Part model, mm, in its own coordinate system. Face numbers are marked on the shaded views. A direction names the side the tool comes from. Give positions to 0.01 mm unless a question says otherwise; leave off trailing zeros. Order: outer loops, then holes, each group sorted by start corner. A loop starts at its lowest first (then second) coordinate and runs counter-clockwise, first axis right, second up.
1. Mould opens along X. For the marked faces 1, 2 and 3 say: +X half, -X half, draft (parallel to the pull), parting line (faces both ways), or undercut.
2. Probe line 1 (Z direction, x = 16.5, y = 2); line 2 (X direction, y = 6, z = 0.2); line 3 (Y direction, x = 28, z = 0.1). List the from-to ranges inside material, lowest first.
3. Slice it at D-D on x = 27. List the corners of the cut face in (y, z), and give its area (3 significant figures).
4. Slice it at C-C on x = 4.5. List the corners of the cut face in (y, z).
5. Slice it at B-B on z = 0.1. List the corners of the cut face in (x, y), and give its area (3 significant figures).
6. Slice it at A-A on x = -10. List the corners of the cut face in (y, z).
7. Which spindle directions (+Z, -Z, +X, -X, +Y, -Y) get a long thin tool onto all of the face, cutting with end or side? Do the marked faces 4 and 5. Say none if no direction does.
Autodesk Inventor part; units mm, degrees
ref_plane "aluschild_XY" through (0, 0, 0) normal (0, 0, 1) x (1, 0, 0)
ref_plane "aluschild_YZ" through (0, 0, 0) normal (1, 0, 0) x (0, 1, 0)
ref_plane "aluschild_ZX" through (0, 0, 0) normal (0, 1, 0) x (0, 0, 1)
sketch "Sketch_1" plane through (0, 0, 0) normal (0, 0, 1) x (1, 0, 0)
  arc A0 (-32, 0) -> (-24, -8) centre (-24, 0) ccw
  line L0 (-24, -8) -> (24, -8)
  arc A1 (24, -8) -> (32, 0) centre (24, 0) ccw
  arc A2 (32, 0) -> (24, 8) centre (24, 0) ccw
  line L1 (24, 8) -> (-24, 8)
  arc A3 (-24, 8) -> (-32, 0) centre (-24, 0) ccw
extrude "Extrusion1" add sketch "Sketch_1" along normal blind 0.3
sketch "Sketch_13" plane through (0, 0, 0.3) normal (0, 0, 1) x (1, 0, 0)
  line L0 (-12.9184, 3.0554) -> (-12.9184, -3.0496)
  line L1 (-12.9184, -3.0496) -> (-10.8856, -3.0496)
  line L2 (-10.8856, -3.0496) -> (-10.8856, -0.7401)
  line L3 (-10.8856, -0.7401) -> (-8.6487, -0.7401)
  line L4 (-8.6487, -0.7401) -> (-8.6487, -3.0496)
  line L5 (-8.6487, -3.0496) -> (-6.6154, -3.0496)
  line L6 (-6.6154, -3.0496) -> (-6.6154, 3.0554)
  line L7 (-6.6154, 3.0554) -> (-8.6487, 3.0554)
  line L8 (-8.6487, 3.0554) -> (-8.6487, 0.8356)
  line L9 (-8.6487, 0.8356) -> (-10.8856, 0.8356)
  line L10 (-10.8856, 0.8356) -> (-10.8856, 3.0554)
  line L11 (-10.8856, 3.0554) -> (-12.9184, 3.0554)
extrude "Extrusion2" cut sketch "Sketch_13" against normal blind 0.05
sketch "Sketch_15" plane through (0, 0, 0.3) normal (0, 0, 1) x (1, 0, 0)
  line L0 (0.5704, 3.0554) -> (0.5704, -3.0496)
  line L1 (0.5704, -3.0496) -> (2.5185, -3.0496)
  line L2 (2.5185, -3.0496) -> (2.5185, 0.0838)
  line L3 (2.5185, 0.0838) -> (5.4533, -3.0496)
  line L4 (5.4533, -3.0496) -> (7.188, -3.0496)
  line L5 (7.188, -3.0496) -> (7.188, 3.0554)
  line L6 (7.188, 3.0554) -> (5.2404, 3.0554)
  line L7 (5.2404, 3.0554) -> (5.2404, -0.0774)
  line L8 (5.2404, -0.0774) -> (2.3062, 3.0554)
  line L9 (2.3062, 3.0554) -> (0.5704, 3.0554)
extrude "Extrusion3" cut sketch "Sketch_15" against normal blind 0.05
sketch "Sketch_16" plane through (0, 0, 0.3) normal (0, 0, 1) x (1, 0, 0)
  line L0 (7.711, 3.0554) -> (7.711, -3.0496)
  line L1 (7.711, -3.0496) -> (9.7438, -3.0496)
  line L2 (9.7438, -3.0496) -> (9.7438, -0.1709)
  line L3 (9.7438, -0.1709) -> (11.8624, -3.0496)
  line L4 (11.8624, -3.0496) -> (14.2863, -3.0496)
  line L5 (14.2863, -3.0496) -> (11.836, 0.2174)
  line L6 (11.836, 0.2174) -> (14.201, 3.0554)
  line L7 (14.201, 3.0554) -> (12.0659, 3.0554)
  line L8 (12.0659, 3.0554) -> (9.7438, 0.2895)
  line L9 (9.7438, 0.2895) -> (9.7438, 3.0554)
  line L10 (9.7438, 3.0554) -> (7.711, 3.0554)
extrude "Extrusion4" cut sketch "Sketch_16" against normal blind 0.05
sketch "Sketch_5" plane through (0, 0, 0.3) normal (0, 0, 1) x (1, 0, 0)
  arc A0 (-22.8125, 0.7425) -> (-21.4625, -0.6075) centre (-21.4625, 0.7425) ccw
  line L0 (-21.4625, -0.6075) -> (-20.7538, -0.6075)
  arc A1 (-20.7538, -1.755) -> (-20.7538, -0.6075) centre (-20.7538, -1.1812) ccw
  line L1 (-20.7538, -1.755) -> (-22.8125, -1.755)
  line L2 (-22.8125, -1.755) -> (-22.8125, -3.0375)
  line L3 (-22.8125, -3.0375) -> (-20.6525, -3.0375)
  arc A2 (-20.6525, -3.0375) -> (-18.7625, -1.1475) centre (-20.6525, -1.1475) ccw
  line L4 (-18.7625, -1.1475) -> (-18.7625, -0.7425)
  arc A3 (-18.7625, -0.7425) -> (-20.1125, 0.6075) centre (-20.1125, -0.7425) ccw
  line L5 (-20.1125, 0.6075) -> (-20.7538, 0.6075)
  arc A4 (-20.7538, 1.755) -> (-20.7538, 0.6075) centre (-20.7358, 1.1812) ccw
  line L6 (-20.7538, 1.755) -> (-18.7625, 1.755)
  line L7 (-18.7625, 1.755) -> (-18.7625, 3.0375)
  line L8 (-18.7625, 3.0375) -> (-20.9225, 3.0375)
  arc A5 (-20.9225, 3.0375) -> (-22.8125, 1.1475) centre (-20.9225, 1.1475) ccw
  line L9 (-22.8125, 1.1475) -> (-22.8125, 0.7425)
extrude "Extrusion5" cut sketch "Sketch_5" against normal blind 0.05
sketch "Sketch_6" plane through (0, 0, 0.3) normal (0, 0, 1) x (1, 0, 0)
  arc A0 (-15.3, 3.0713) -> (-15.3, -3.0713) centre (-15.3, 0) ccw
  line L0 (-15.3, -3.0713) -> (-13.545, -3.0713)
  line L1 (-13.545, -3.0713) -> (-13.545, -1.1475)
  line L2 (-13.545, -1.1475) -> (-15.3, -1.1475)
  arc A1 (-15.3, 1.1475) -> (-15.3, -1.1475) centre (-15.3, 0) ccw
  line L3 (-15.3, 1.1475) -> (-13.545, 1.1475)
  line L4 (-13.545, 1.1475) -> (-13.545, 3.0713)
  line L5 (-13.545, 3.0713) -> (-15.3, 3.0713)
extrude "Extrusion6" cut sketch "Sketch_6" against normal blind 0.05
sketch "Sketch_7" plane through (0, 0, 0.3) normal (0, 0, 1) x (1, 0, 0)
  line L0 (-6.04, 2.97) -> (-6.04, 0)
  arc A0 (-6.04, 0) -> (0.035, 0) centre (-3.0025, 0) ccw
  line L1 (0.035, 0) -> (0.035, 2.97)
  line L2 (0.035, 2.97) -> (-1.9225, 2.97)
  line L3 (-1.9225, 2.97) -> (-1.9225, 0)
  arc A1 (-4.0825, 0) -> (-1.9225, 0) centre (-3.0025, 0) ccw
  line L4 (-4.0825, 0) -> (-4.0825, 2.97)
  line L5 (-4.0825, 2.97) -> (-6.04, 2.97)
extrude "Extrusion7" cut sketch "Sketch_7" against normal blind 0.05
sketch "Sketch8" plane through (0, 0, 0.3) normal (0, 0, 1) x (1, 0, 0)
  point P0 (20, 0)
hole "Hole1" at (20, 0, 0.3) direction (0, 0, -1) diameter 2.832 depth 0.05
sketch "Sketch_3" plane through (0, 0, 0.3) normal (0, 0, 1) x (1, 0, 0)
  arc A0 (21.4558, 4.7829) -> (15.4894, -2.1564) centre (20, 0) ccw
  line L0 (15.4894, -2.1564) -> (18.1798, -0.7416)
  arc A1 (21.6256, 1.1048) -> (18.1798, -0.7416) centre (20, 0) ccw
  line L1 (21.6256, 1.1048) -> (24.9442, 2.8689)
  line L2 (24.9442, 2.8689) -> (24.9442, 6.6331)
  line L3 (24.9442, 6.6331) -> (21.4558, 4.7829)
extrude "Extrusion8" cut sketch "Sketch_3" against normal blind 0.05
sketch "Sketch_4" plane through (0, 0, 0.3) normal (0, 0, 1) x (1, 0, 0)
  line L0 (15.0735, -2.8571) -> (15.0735, -6.6213)
  line L1 (15.0735, -6.6213) -> (18.5633, -4.7863)
  arc A0 (18.5633, -4.7863) -> (24.4981, 2.1771) centre (20, 0) ccw
  line L2 (24.4981, 2.1771) -> (21.8157, 0.7331)
  arc A1 (18.3864, -1.1091) -> (21.8157, 0.7331) centre (20, 0) ccw
  line L3 (18.3864, -1.1091) -> (15.0735, -2.8571)
extrude "Extrusion9" cut sketch "Sketch_4" against normal blind 0.05
ref_plane "aluschild_XY" through (0, 0, 0) normal (0, 0, 1) x (1, 0, 0)
ref_plane "aluschild_YZ" through (0, 0, 0) normal (1, 0, 0) x (0, 1, 0)
ref_plane "aluschild_ZX" through (0, 0, 0) normal (0, 1, 0) x (0, 0, 1)
properties part number "SCHUNK-9957615 Typenschild 16x64x0.3"
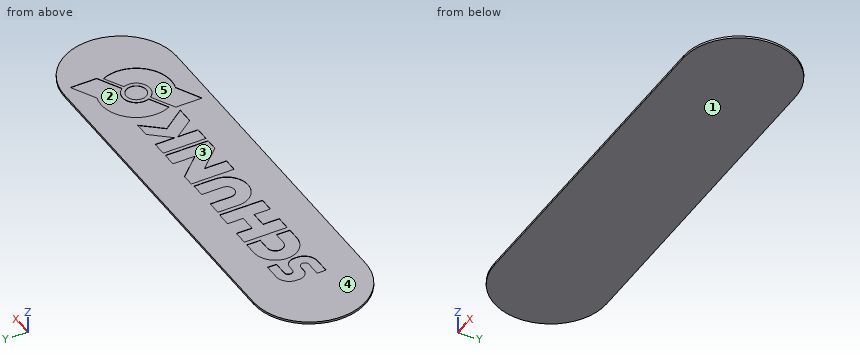
Data:
1. face 1: draft
1. face 2: undercut
1. face 3: undercut
2. line 1: z = 0 to 0.25
2. line 2: x = -29.29 to 29.29
2. line 3: y = -6.93 to 6.93
3. outline: (-7.42, 0) - (7.42, 0) - (7.42, 0.3) - (-7.42, 0.3) - close
3. area: 4.45 mm2
4. outline: (-8, 0) - (8, 0) - (8, 0.3) - (0.71, 0.3) - (0.71, 0.25) - (-2.03, 0.25) - (-2.03, 0.3) - (-8, 0.3) - close
5. outline: (-24, -8) - (24, -8) arc R8 ccw to (24, 8) - (-24, 8) arc R8 ccw to start
5. area: 969 mm2
6. outline: (-8, 0) - (8, 0) - (8, 0.3) - (0.84, 0.3) - (0.84, 0.25) - (-0.74, 0.25) - (-0.74, 0.3) - (-8, 0.3) - close
7. face 4: +Z, +X, -X, +Y, -Y
7. face 5: +Z
